Source: three-view drawing plus pictorial views. Frame: mm from the lowest corner of the part. A direction names the side the tool comes from. Give positions to 0.01 mm unless a question says otherwise; leave off trailing zeros. Write each loop counter-clockwise with the first axis right and the second up, starting at its lowest first coordinate (ties: lowest second). Pieces come first, ordered by that corner, then holes. Notation, with made-up numbers: M 52.5,-39 L 99.5,-39 A23 ccw 99.5,-26 Z; hole C -18,30 d10. An arc over 180 degrees is marked long. One line per question, with ' | ' between items.
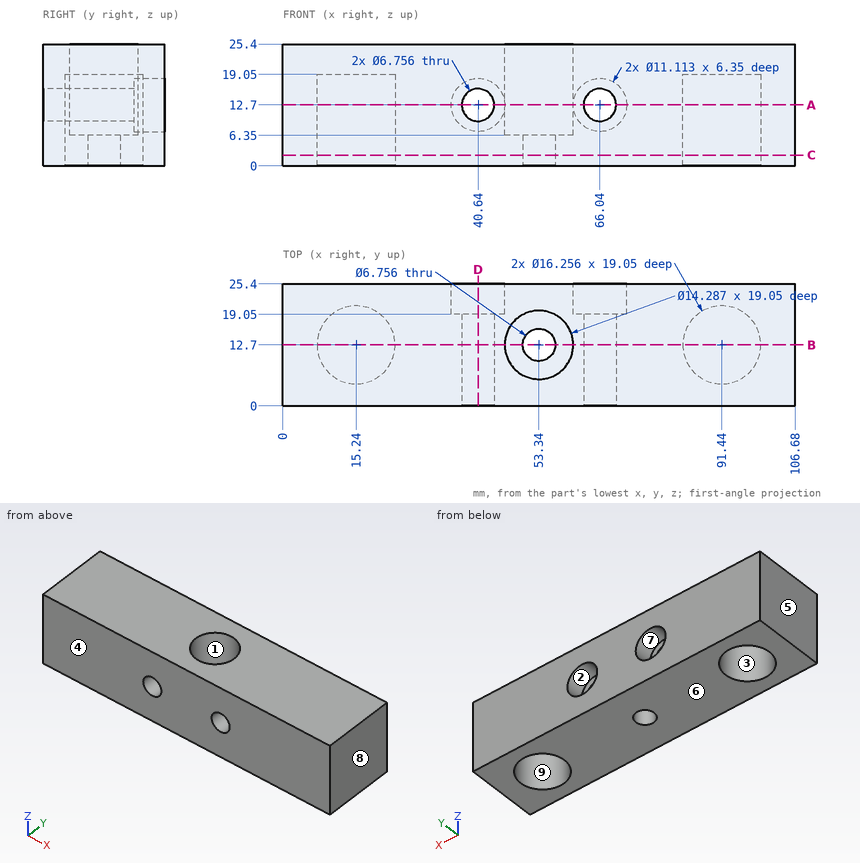
(1) Cut plane D-D, the plane x = 40.64. Return loops of the section in (y, z), then the cut area to 3 significant figures.
Working result:
outline: M 0,0 L 25.4,0 L 25.4,7.14 L 19.05,7.14 L 19.05,9.32 L 0,9.32 Z; M 0,16.08 L 19.05,16.08 L 19.05,18.26 L 25.4,18.26 L 25.4,25.4 L 0,25.4 Z | area: 446 mm^2
(2) Draft query along X for the marked faces 6, 7, 8 and 9. Return one class per face: released by +X, released by -X, zero draft, split by the parting line, or undercut.
Working result:
face 6: zero draft | face 7: undercut | face 8: released by +X | face 9: undercut
(3) First-contact query: P1, Ø8, axis at x = 89.5, y = 16, coming from the -Z side; P2, Ø5.5, axis at x = 41, z = 14.5, coming from the +Y side; P3, Ø6, axis at x = 53.34, y = 12.7, coming from the -Z side. Flat tips, straight axial feed; report the tip coordinate or a pass-through.
Working result:
P1: stops at z = 19.05 | P2: stops at y = 19.05 | P3: passes through
(4) Cut plane A-A, the plane z = 12.7. Count the separate pieces of the cut face and the enclosed holes in it, then the cut area to 3 significant figures.
Working result:
separate pieces: 3 | enclosed holes: 3 | area: 1,740 mm^2
(5) Cut plane B-B, the plane y = 12.7. Return loops of the section in (x, z).
Working result:
outline: M 0,0 L 7.11,0 L 7.11,19.05 L 23.37,19.05 L 23.37,0 L 49.96,0 L 49.96,6.35 L 46.2,6.35 L 46.2,25.4 L 0,25.4 Z; M 56.72,0 L 83.31,0 L 83.31,19.05 L 99.57,19.05 L 99.57,0 L 106.68,0 L 106.68,25.4 L 60.48,25.4 L 60.48,6.35 L 56.72,6.35 Z; hole C 40.64,12.7 d6.76; hole C 66.04,12.7 d6.76
(6) Cut plane C-C, the plane z = 2.25. Return loops of the section in (x, y) (1 decimal), then the cut area to 3 significant figures.
Working result:
outline: M 0,0 L 106.7,0 L 106.7,25.4 L 0,25.4 Z; hole C 15.2,12.7 d16.3; hole C 53.3,12.7 d6.8; hole C 91.4,12.7 d16.3 | area: 2,260 mm^2
(7) Material intervals for L1, parallel to X at y = 13, z = 12.7; L2, parallel to Y at x = 53.34, z = 19; L3, parallel to X at y = 2.5, z = 15 (1 decimal), sorted ascending. Write a range as [from, to].
Working result:
L1: x = [0, 7.12], [23.36, 37.26], [44.02, 46.2], [60.48, 62.66], [69.42, 83.32], [99.56, 106.68] | L2: y = [0, 5.56], [19.84, 25.4] | L3: x = [0, 38.2], [43.1, 63.6], [68.5, 106.7]
(8) Set-up query: the marked faces 1, 2, 3, 4 and 5. Return all of +Z, -Z, +X, -X, +Y, -Y with unobstructed straight access to the full face (end or side cutting, diameter ignored); none if empty.
Working result:
face 1: +Z | face 2: +Y | face 3: -Z | face 4: +Z, -Z, +X, -X, -Y | face 5: +Z, -Z, -X, +Y, -Y
